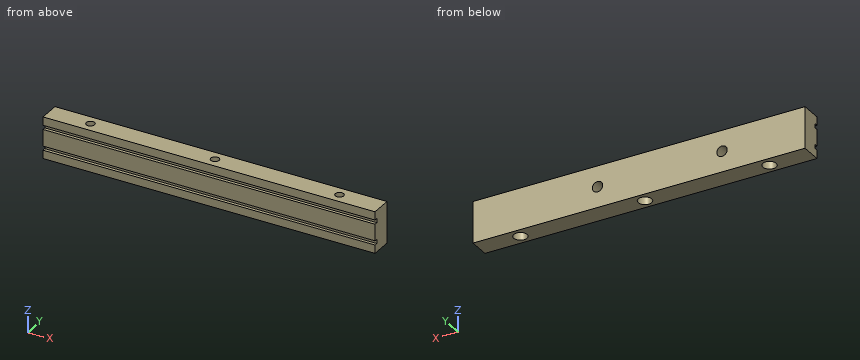
from build123d import *

# Parameters (mm, degrees)
IZIM1_W                                      = 160
IZIM1_H                                      = 10
Y_KSEKLIK_EKSTR_ZYON1_DEPTH                  = 20
F_4_0MM_SAPLAMA_DELIKLERI1_D                 = 5
F_4_0MM_SAPLAMA_DELIKLERI1_DEPTH             = 8
IZIM6_W                                      = 2
IZIM6_H                                      = 1.5
KES_EKSTR_ZYON1_DEPTH                        = 162.554944214
M5_ALT_GEN_BA_L_C_VATA_IN_HAV_A1_D           = 4
M5_ALT_GEN_BA_L_C_VATA_IN_HAV_A1_CBORE_D     = 6.5
M5_ALT_GEN_BA_L_C_VATA_IN_HAV_A1_CBORE_DEPTH = 6


with BuildPart() as part:
    # Çizim1 → Yükseklik-Ekstrüzyon1 (new body)
    with BuildSketch(Plane.XY):
        with Locations((80, 5)):
            Rectangle(IZIM1_W, IZIM1_H)
    extrude(amount=Y_KSEKLIK_EKSTR_ZYON1_DEPTH)

    # Ø4.0mm Saplama Delikleri1
    with Locations(Plane(origin=(40, 10, 10), x_dir=(0, 0, 1), z_dir=(0, 1, 0))):
        with Locations((0, 0), (0, 60)):
            Hole(F_4_0MM_SAPLAMA_DELIKLERI1_D / 2, depth=F_4_0MM_SAPLAMA_DELIKLERI1_DEPTH)

    # Çizim6 → Kes-Ekstrüzyon1 (cut, through all)
    with BuildSketch(Plane.ZY):
        with Locations((5, 0.75)):
            Rectangle(IZIM6_W, IZIM6_H)
        with Locations((15, 0.75)):
            Rectangle(IZIM6_W, IZIM6_H)
    extrude(amount=-KES_EKSTR_ZYON1_DEPTH, mode=Mode.SUBTRACT)

    # M5 Altıgen Başlı Cıvata İçin Havşa1 (through all)
    with Locations(Plane(origin=(140, 5, 0), x_dir=(-1, 0, 0), z_dir=(0, 0, -1))):
        with Locations((0, 0), (60, 0), (120, 0)):
            CounterBoreHole(M5_ALT_GEN_BA_L_C_VATA_IN_HAV_A1_D / 2, M5_ALT_GEN_BA_L_C_VATA_IN_HAV_A1_CBORE_D / 2, M5_ALT_GEN_BA_L_C_VATA_IN_HAV_A1_CBORE_DEPTH)


solid = part.part
Check sheet for the modelled part. Datum: model origin and axes. Units: mm. Coordinates: 2 decimals unless noted, no trailing zeros. Loops run counter-clockwise (first coordinate to the right, second up) from the corner with the lowest first, then second, coordinate; pieces in that order, holes last. Notation, with made-up numbers: (8.25, 11.5) -> (24.25, 11.5) arc R20 cw to (24.25, 40.5) -> close; hole circle Ø8 at (42.25, 22.5). An arc over 180 degrees is marked (long way). Answer in a Markdown table with one row per item.
1. Material ranges on line 1 along Y through (x, z) = (80, 1.5); line 2 along Y through (x, z) = (140, 10); line 3 along Z through (x, y) = (93.5, 1), recorded low to high. Write a range as [from, to].
Check values:
| item | result |
|---|---|
| line 1 | y = [0, 1.75], [8.25, 10] |
| line 2 | y = [0, 3], [7, 10] |
| line 3 | z = [0, 4], [6, 14], [16, 20] |
2. Go/stop test with flat-tipped pins: pin 1 (0.6 mm diameter, centred on x = 54, z = 5, fed in from -Y); pin 2 (5 mm diameter, centred on x = 80, y = 5, fed in from -Z); pin 3 (1.5 mm diameter, centred on x = 39, z = 11, fed in from +Y). Record where each tip stops, or that it passes through.
Check values:
| item | result |
|---|---|
| pin 1 | stops at y = 1.5 |
| pin 2 | stops at z = 6 |
| pin 3 | stops at y = 2 |
3. Sectioned sample at B-B, the plane x = 140. Record the boundary of the cut face in (y, z), then the cut area to 3 significant figures.
Check values:
| item | result |
|---|---|
| outline | (0, 0) -> (1.75, 0) -> (1.75, 6) -> (3, 6) -> (3, 20) -> (0, 20) -> (0, 16) -> (1.5, 16) -> (1.5, 14) -> (0, 14) -> (0, 6) -> (1.5, 6) -> (1.5, 4) -> (0, 4) -> close; (7, 6) -> (8.25, 6) -> (8.25, 0) -> (10, 0) -> (10, 20) -> (7, 20) -> close |
| area | 99.0 mm2 |
4. Sectioned sample at C-C, the plane x = 117. Record the boundary of the cut face in (y, z).
Check values:
| item | result |
|---|---|
| outline | (0, 0) -> (10, 0) -> (10, 20) -> (0, 20) -> (0, 16) -> (1.5, 16) -> (1.5, 14) -> (0, 14) -> (0, 6) -> (1.5, 6) -> (1.5, 4) -> (0, 4) -> close |
5. Sectioned sample at A-A, the plane y = 5. Give the number of separate pieces and of enclosed holes in the cut face, then the cut area to 3 significant figures.
Check values:
| item | result |
|---|---|
| separate pieces | 4 |
| enclosed holes | 2 |
| area | 2,880 mm2 |
6. Sectioned sample at D-D, the plane x = 40. Record the boundary of the cut face in (y, z).
Check values:
| item | result |
|---|---|
| outline | (0, 0) -> (10, 0) -> (10, 7.5) -> (2, 7.5) -> (2, 12.5) -> (10, 12.5) -> (10, 20) -> (0, 20) -> (0, 16) -> (1.5, 16) -> (1.5, 14) -> (0, 14) -> (0, 6) -> (1.5, 6) -> (1.5, 4) -> (0, 4) -> close |
